The listing builds one solid part. Answer for the finished solid, in the listing's coordinates (mm). Coordinates: 2 decimals unless noted, no trailing zeros. Answer as CSV lines item,"result".
```python
from build123d import *

# Parameters (mm, degrees)
BOSS_EXTRUDE1_DEPTH  = 2
SKETCH2_R            = 2.028178019
CUT_EXTRUDE1_DEPTH   = 2
LPATTERN1_COUNT      = 6
LPATTERN1_PITCH      = 4.5
LPATTERN2_COUNT      = 8
LPATTERN2_PITCH      = 4.5
SKETCH4_R            = 2
CUT_EXTRUDE3_DEPTH   = 2
LPATTERN4_COUNT      = 8
LPATTERN4_PITCH      = 4.5
LPATTERN4_COUNT_DIR2 = 6
LPATTERN4_PITCH_DIR2 = 4.5
SKETCH5_R            = 2
CUT_EXTRUDE4_DEPTH   = 2
LPATTERN5_COUNT      = 6
LPATTERN5_PITCH      = 4.5
LPATTERN5_COUNT_DIR2 = 6
LPATTERN5_PITCH_DIR2 = 4.5
SKETCH6_W            = 0.774823081
SKETCH6_H            = 1.866619241
CUT_EXTRUDE5_DEPTH   = 3
SKETCH7_R            = 2
CUT_EXTRUDE6_DEPTH   = 3
LPATTERN6_DEPTH      = 2
LPATTERN7_COUNT      = 2
LPATTERN7_PITCH      = 4.5
SKETCH8_R            = 5
CUT_EXTRUDE7_DEPTH   = 10


# Read off the part's stored shape, not the designer's step: LPattern6
with BuildPart() as part:
    # Sketch1 → Boss-Extrude1 (new body)
    with BuildSketch(Plane(origin=(0, 0, 0), x_dir=(1, 0, 0), z_dir=(0, 1, 0))):
        Polygon((-12.273533446, 20.252933108), (12.726466554, 20.252933108), (30.226466554, -8.897066892), (23.726466554, -19.347066892), (-23.273533446, -19.347066892), (-29.773533446, -8.897066892), align=None)
    extrude(amount=BOSS_EXTRUDE1_DEPTH)

    # Sketch2 → Cut-Extrude1 (cut)
    with BuildSketch(Plane(origin=(0, 2, 0), x_dir=(1, 0, 0), z_dir=(0, 1, 0))):
        with Locations(Location((11.377256113, 17.701051842, 0), (0, 0, 270))):
            Circle(SKETCH2_R)
    cut_extrude1 = extrude(amount=-CUT_EXTRUDE1_DEPTH, mode=Mode.SUBTRACT)

    # LPattern1: Cut-Extrude1 ×6
    with Locations(*[(-i * LPATTERN1_PITCH, 0, 0) for i in range(1, LPATTERN1_COUNT)]):
        add(cut_extrude1, mode=Mode.SUBTRACT)

    # LPattern2: Cut-Extrude1 ×8
    with Locations(*[Vector(0.5147120046125901, 0, 0.8573631391118288) * (i * LPATTERN2_PITCH) for i in range(1, LPATTERN2_COUNT)]):
        add(cut_extrude1, mode=Mode.SUBTRACT)

    # Sketch4 → Cut-Extrude3 (cut)
    with BuildSketch(Plane(origin=(0, 2, 0), x_dir=(1, 0, 0), z_dir=(0, 1, 0))):
        with Locations(Location((9.248601258, 13.393901657, 0), (0, 0, 270))):
            Circle(SKETCH4_R)
    cut_extrude3 = extrude(amount=-CUT_EXTRUDE3_DEPTH, mode=Mode.SUBTRACT)

    # LPattern4: Cut-Extrude3 8 × 6
    with Locations(*[Vector(0.5147120046125901, 0, 0.8573631391118288) * (i * LPATTERN4_PITCH) + Vector(-1, 0, 0) * (j * LPATTERN4_PITCH_DIR2) for i in range(LPATTERN4_COUNT) for j in range(LPATTERN4_COUNT_DIR2) if (i, j) != (0, 0)]):
        add(cut_extrude3, mode=Mode.SUBTRACT)

    # Sketch5 → Cut-Extrude4 (cut)
    with BuildSketch(Plane(origin=(0, 2, 0), x_dir=(1, 0, 0), z_dir=(0, 1, 0))):
        with Locations(Location((-15.435194721, 9.535767531, 0), (0, 0, 270))):
            Circle(SKETCH5_R)
    cut_extrude4 = extrude(amount=-CUT_EXTRUDE4_DEPTH, mode=Mode.SUBTRACT)

    # LPattern5: Cut-Extrude4 6 × 6
    with Locations(*[Vector(-0.5147120046125901, 0, 0.8573631391118288) * (i * LPATTERN5_PITCH) + Vector(0.5147120046125901, 0, 0.8573631391118288) * (j * LPATTERN5_PITCH_DIR2) for i in range(LPATTERN5_COUNT) for j in range(LPATTERN5_COUNT_DIR2) if (i, j) != (0, 0)]):
        add(cut_extrude4, mode=Mode.SUBTRACT)

    # Sketch6 → Cut-Extrude5 (cut)
    with BuildSketch(Plane(origin=(0, 2, 0), x_dir=(1, 0, 0), z_dir=(0, 1, 0))):
        with Locations((-23.405230337, -19.594174878)):
            Rectangle(SKETCH6_W, SKETCH6_H)
    extrude(amount=-CUT_EXTRUDE5_DEPTH, mode=Mode.SUBTRACT)

    # Sketch7 → Cut-Extrude6 (cut)
    with BuildSketch(Plane(origin=(0, 2, 0), x_dir=(1, 0, 0), z_dir=(0, 1, 0))):
        with Locations((-3.986582659, -17.471171351)):
            Circle(SKETCH7_R)
    cut_extrude6 = extrude(amount=-CUT_EXTRUDE6_DEPTH, mode=Mode.SUBTRACT)

    # LPattern6 outline → LPattern6 (cut)
    with BuildSketch(Plane(origin=(0, 0, 0), x_dir=(1, 0, 0), z_dir=(0, 1, 0))):
        with BuildLine():
            Line((-0.180135771, -19.347066892), (1.206970453, -19.347066892))
            ThreePointArc((1.206970453, -19.347066892), (0.513417341, -15.471171351), (-0.180135771, -19.347066892))
        make_face()
        with BuildLine():
            ThreePointArc((25.00529483, -17.291104509), (21.79762259, -15.883140142), (22.319864229, -19.347066892))
            Line((22.319864229, -19.347066892), (23.726466554, -19.347066892))
            Line((23.726466554, -19.347066892), (25.00529483, -17.291104509))
        make_face()
        with BuildLine():
            ThreePointArc((19.206970453, -19.347066892), (18.513417341, -15.471171351), (17.819864229, -19.347066892))
            Line((17.819864229, -19.347066892), (19.206970453, -19.347066892))
        make_face()
        with BuildLine():
            ThreePointArc((14.706970453, -19.347066892), (14.013417341, -15.471171351), (13.319864229, -19.347066892))
            Line((13.319864229, -19.347066892), (14.706970453, -19.347066892))
        make_face()
        with BuildLine():
            ThreePointArc((10.206970453, -19.347066892), (9.513417341, -15.471171351), (8.819864229, -19.347066892))
            Line((8.819864229, -19.347066892), (10.206970453, -19.347066892))
        make_face()
        with BuildLine():
            ThreePointArc((5.706970453, -19.347066892), (5.013417341, -15.471171351), (4.319864229, -19.347066892))
            Line((4.319864229, -19.347066892), (5.706970453, -19.347066892))
        make_face()
    extrude(amount=LPATTERN6_DEPTH, mode=Mode.SUBTRACT)

    # LPattern7: Cut-Extrude6 ×2
    with Locations(*[Vector(0.5281717070926116, 0, -0.8491375906335066) * (i * LPATTERN7_PITCH) for i in range(1, LPATTERN7_COUNT)]):
        add(cut_extrude6, mode=Mode.SUBTRACT)

    # Sketch8 → Cut-Extrude7 (cut)
    with BuildSketch(Plane(origin=(0, 2, 0), x_dir=(1, 0, 0), z_dir=(0, 1, 0))):
        Circle(SKETCH8_R)
    extrude(amount=-CUT_EXTRUDE7_DEPTH, mode=Mode.SUBTRACT)


solid = part.part
```
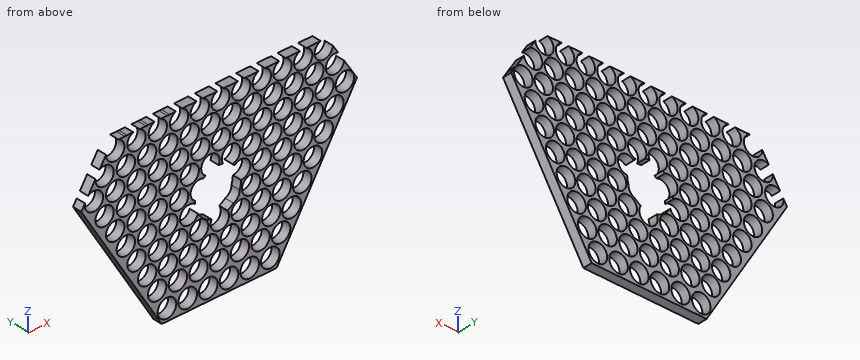
Q1. Find section A-A (z = -14). Count the separate pieces of the cut face and the enclosed holes in it, and give its area (3 significant figures).
Output:
separate pieces,"8"
enclosed holes,"0"
area,"11.2 mm2"
Q2. Straight lines are drawn through the part: line 1 (Z direction, x = 26, y = 1.7); line 2 (Z direction, x = -23, y = 1.4). For each, find the intervals that lie inside material, in ascending order.
Output:
line 1,"1.86 to 3.55, 7.34 to 8.05, 10.56 to 11.69, 15.54 to 15.69"
line 2,"-2.39 to 0.14, 3.94 to 4.84, 6.95 to 7.85, 11.66 to 12.56, 14.67 to 15.57"
Q3. Flat-ended cylindrical pins translate along their axes: pin 1 Ø3.5 at (x, z) = (18.51, 2.04) entering from +Y; pin 2 Ø6.5 at (x, z) = (-8.62, -5.68) entering from -Y. Find the tip coordinate at first contact, or state that the pin passes through.
Output:
pin 1,"through"
pin 2,"y = 0"
